CAD build for the part. Positions are in the model's coordinates, mm. A direction names the side the tool comes from. Round coordinates to 2 decimals unless told otherwise and drop trailing zeros. Write each loop counter-clockwise with the first axis right and the second up, starting at its lowest first coordinate (ties: lowest second). Pieces come first, ordered by that corner, then holes. Notation, with made-up numbers: (73.25, 58) -> (89.25, 58) arc R16 cw to (89.25, 82) -> close; hole circle Ø4 at (62, 49). An arc over 180 degrees is marked (long way). Put each result on its own line as item: value. Start each with the question number.
1. Flat gauge pins, fed straight in: P1, Ø1, axis at x = 143, y = 21.5, coming from the -Z side; P2, Ø1, axis at x = 146, z = -25.5, coming from the +Y side; P3, Ø1.1, axis at y = 22.5, z = -1.5, coming from the -X side. Where does each tip first touch, or does it go through?
2. 3-axis set-ups, long thin cutter, end or side, ignore diameter. For faces 1 (the flat face through (143, 22, -1)), 2 (the flat face through (168, 11, -30)), 3 (the flat face through (143, 22, -60)): which of +Z, -Z, +X, -X, +Y, -Y reach the whole face in a straight line?
3. Saw through at D-D on y = 6.5. List the corners of the cut face in (x, z).
4. Saw through at A-A on x = 142. List the corners of the cut face in (y, z), and give its area (3 significant figures).
5. Saw through at C-C on y = 14.25. List the corners of the cut face in (x, z) (3 decimals), and give its area (3 significant figures).
6. Saw through at B-B on z = -5. List the corners of the cut face in (x, y).
7. Pull direction Z, two halves, no side cores. Call faces 4 (the flat face through (27, 22, -1)), 5 (the flat face through (27, 22, -60)), 6 (the flat face through (84, 12, -59)): pulls with the +Z half, pulls with the -Z half, needs draft (parallel to the pull), parting line crosses it, or undercut.
8. Drill centre lines: line 1 (X direction, y = 5.75, z = -49.5); line 2 (Z direction, x = 8, y = 13.25); line 3 (Y direction, x = 151, z = -37.5). Where is each one in solid material? Low to high. Write a range as from..to.
from build123d import *

# Parameters (mm, degrees)
SKETCH1_W           = 170
SKETCH1_H           = 61
BOSS_EXTRUDE1_DEPTH = 20
SKETCH2_W           = 166
SKETCH2_H           = 57
CUT_EXTRUDE1_DEPTH  = 18
SKETCH3_W           = 10
SKETCH3_H           = 1
BOSS_EXTRUDE2_DEPTH = 6
CUT_EXTRUDE2_DEPTH  = 200
SKETCH5_W           = 10.85
SKETCH5_H           = 8
CUT_EXTRUDE3_DEPTH  = 5


with BuildPart() as part:
    # Sketch1 → Boss-Extrude1 (new body)
    with BuildSketch(Plane(origin=(0, 0, 0), x_dir=(1, 0, 0), z_dir=(0, 1, 0))):
        with Locations((85, 30.5)):
            Rectangle(SKETCH1_W, SKETCH1_H)
    extrude(amount=BOSS_EXTRUDE1_DEPTH)

    # Sketch2 → Cut-Extrude1 (cut)
    with BuildSketch(Plane(origin=(0, 20, 0), x_dir=(1, 0, 0), z_dir=(0, 1, 0))):
        with Locations((85, 30.5)):
            Rectangle(SKETCH2_W, SKETCH2_H)
    extrude(amount=-CUT_EXTRUDE1_DEPTH, mode=Mode.SUBTRACT)

    # Sketch3 → Boss-Extrude2 (add)
    with BuildSketch(Plane(origin=(0, 20, 0), x_dir=(1, 0, 0), z_dir=(0, 1, 0))):
        with Locations((27, 1.5)):
            Rectangle(SKETCH3_W, SKETCH3_H)
        with Locations((143, 1.5)):
            Rectangle(SKETCH3_W, SKETCH3_H)
        with Locations((27, 59.5)):
            Rectangle(SKETCH3_W, SKETCH3_H)
        with Locations((143, 59.5)):
            Rectangle(SKETCH3_W, SKETCH3_H)
    extrude(amount=BOSS_EXTRUDE2_DEPTH)

    # Sketch4 → Cut-Extrude2 (cut)
    with BuildSketch(Plane.ZY.offset(-22)):
        Polygon((-60, 25), (-59, 26), (-60, 26), align=None)
        Polygon((-59.646446609, 24.146446609), (-60, 24.5), (-60, 23.292893219), (-59.646446609, 23.646446609), align=None)
        Polygon((-1, 26), (-2, 26), (-1, 25), align=None)
        Polygon((-1, 23.292893219), (-1, 24.5), (-1.353553391, 24.146446609), (-1.353553391, 23.646446609), align=None)
    extrude(amount=-CUT_EXTRUDE2_DEPTH, mode=Mode.SUBTRACT)

    # Sketch5 → Cut-Extrude3 (cut)
    with BuildSketch(Plane.ZY):
        with Locations((-30.5, 16)):
            Rectangle(SKETCH5_W, SKETCH5_H)
    extrude(amount=-CUT_EXTRUDE3_DEPTH, mode=Mode.SUBTRACT)


solid = part.part
Return value:
1. P1: stops at z = -60
1. P2: stops at y = 2
1. P3: stops at x = 22
2. face 1: +Z, +X, -X, +Y
2. face 2: +Y
2. face 3: -Z, +X, -X, +Y
3. outline: (0, -61) -> (170, -61) -> (170, 0) -> (0, 0) -> close; hole (2, -59) -> (168, -59) -> (168, -2) -> (2, -2) -> close
4. outline: (0, -61) -> (20, -61) -> (20, -60) -> (23.29, -60) -> (23.65, -59.65) -> (24.15, -59.65) -> (24.5, -60) -> (25, -60) -> (26, -59) -> (2, -59) -> (2, -2) -> (26, -2) -> (25, -1) -> (24.5, -1) -> (24.15, -1.35) -> (23.65, -1.35) -> (23.29, -1) -> (20, -1) -> (20, 0) -> (0, 0) -> close
4. area: 204 mm^2
5. outline: (0, -61) -> (170, -61) -> (170, 0) -> (0, 0) -> (0, -25.075) -> (2, -25.075) -> (2, -2) -> (168, -2) -> (168, -59) -> (2, -59) -> (2, -35.925) -> (0, -35.925) -> close
5. area: 886 mm^2
6. outline: (0, 0) -> (170, 0) -> (170, 20) -> (168, 20) -> (168, 2) -> (2, 2) -> (2, 20) -> (0, 20) -> close
7. face 4: pulls with the +Z half
7. face 5: pulls with the -Z half
7. face 6: undercut
8. line 1: x = 0..2, 168..170
8. line 2: z = -61..-59, -2..0
8. line 3: y = 0..2
